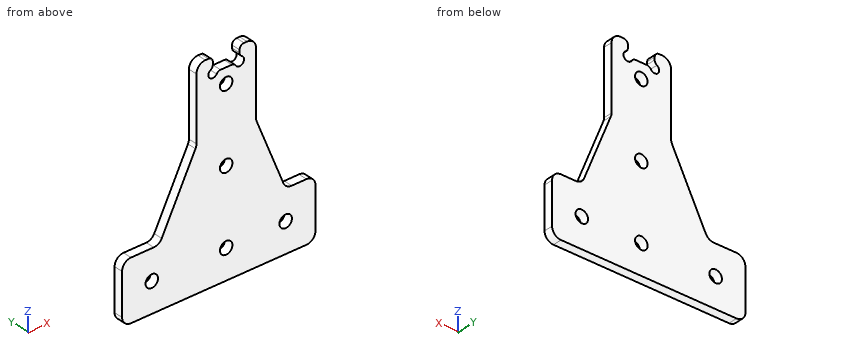
```python
from build123d import *

# Parameters (mm, degrees)
SKETCH_1_R          = 2.1
EXTRUDE_1_DEPTH     = 3
FILLET_1_R          = 3
SKETCH_2_W          = 9
SKETCH_2_H          = 5
CUT_EXTRUDE_1_DEPTH = 3
SKETCH_3_R          = 1.5
CUT_EXTRUDE_2_DEPTH = 10
FILLET_2_R          = 1.5


with BuildPart() as part:
    # 草图1 → 凸台-拉伸1 (new body)
    # profile 1 of 3: a face of its own
    with BuildSketch(Plane(origin=(0, 0, 0), x_dir=(1, 0, 0), z_dir=(0, 1, 0))):
        Polygon((10, -10), (30, -10), (30, 10), (-35, 10), (-35, -10), (-10, -10), (-10, -60), (10, -60), align=None)
        with Locations(Location((0, -50, 0), (0, 0, 270))):
            Circle(SKETCH_1_R, mode=Mode.SUBTRACT)
        with Locations(Location((0, -25, 0), (0, 0, 270))):
            Circle(SKETCH_1_R, mode=Mode.SUBTRACT)
        with Locations(Location((-25, 0, 0), (0, 0, 270))):
            Circle(SKETCH_1_R, mode=Mode.SUBTRACT)
        with Locations(Location((20, 0, 0), (0, 0, 270))):
            Circle(SKETCH_1_R, mode=Mode.SUBTRACT)
        with Locations(Location((0, 0, 0), (0, 0, 270))):
            Circle(SKETCH_1_R, mode=Mode.SUBTRACT)
    # profile 2 of 3: a face of its own
    with BuildSketch(Plane(origin=(0, 0, 0), x_dir=(1, 0, 0), z_dir=(0, 1, 0))):
        Polygon((-10, -10), (-22.5, -10), (-10, -35), align=None)
    # profile 3 of 3: a face of its own
    with BuildSketch(Plane(origin=(0, 0, 0), x_dir=(1, 0, 0), z_dir=(0, 1, 0))):
        Polygon((10, -35), (20, -10), (10, -10), align=None)
    extrude(amount=EXTRUDE_1_DEPTH)

    # 圆角1
    fillet_1_edges = [part.edges().sort_by_distance(p)[0] for p in [
        (10, 1.5, 35),
        (10, 1.5, 60),
        (-10, 1.5, 60),
        (-10, 1.5, 35),
        (-22.5, 1.5, 10),
        (-35, 1.5, 10),
        (-35, 1.5, -10),
        (30, 1.5, -10),
        (30, 1.5, 10),
        (20, 1.5, 10),
    ]]
    fillet(fillet_1_edges, radius=FILLET_1_R)

    # 草图2 → 切除-拉伸1 (cut)
    with BuildSketch(Plane(origin=(0, 3, 0), x_dir=(1, 0, 0), z_dir=(0, 1, 0))):
        with Locations((0, -57.5)):
            Rectangle(SKETCH_2_W, SKETCH_2_H)
    extrude(amount=-CUT_EXTRUDE_1_DEPTH, mode=Mode.SUBTRACT)

    # 草图3 → 切除-拉伸2 (cut)
    with BuildSketch(Plane(origin=(0, 3, 0), x_dir=(1, 0, 0), z_dir=(0, 1, 0))):
        with Locations((-4.5, -55)):
            Circle(SKETCH_3_R)
        with Locations((4.5, -55)):
            Circle(SKETCH_3_R)
    extrude(amount=-CUT_EXTRUDE_2_DEPTH, mode=Mode.SUBTRACT)

    # 圆角2
    fillet_2_edges = [part.edges().sort_by_distance(p)[0] for p in [
        (-4.5, 1.5, 60),
        (4.5, 1.5, 60),
        (4.5, 1.5, 56.5),
        (-3, 1.5, 55),
        (-4.5, 1.5, 56.5),
        (3, 1.5, 55),
    ]]
    fillet(fillet_2_edges, radius=FILLET_2_R)


solid = part.part
```
Can you work these out from the model? Positions are in its coordinate system, mm. Round coordinates to 2 decimals unless told otherwise and drop trailing zeros. Order: outer loops, then holes, each group sorted by start corner. A loop starts at its lowest first (then second) coordinate and runs counter-clockwise, first axis right, second up. Notation, with made-up numbers: (34.25, -4.75) -> (41.25, -4.75) arc R11 ccw to (41.25, 0.25) -> close; hole circle Ø1 at (-14, 63). An arc over 180 degrees is marked (long way). Return JSON: item names as keys, results as strings. Group by question number.
1. If we section it at C-C, the plane y = 1.1: Count the separate pieces of the cut face and the enclosed holes in it, then the cut area to 3 significant figures.
2. If we section it at A-A, the plane z = 0: Write out the boundary of the cut face in (x, y), then the cut area to 3 significant figures.
3. If we section it at D-D, the plane x = 23.5: Write out the boundary of the cut face in (y, z).
4. I need wall thicknesses on line 1 (X direction, y = 1.95, z = 0); line 2 (X direction, y = 2.8, z = 50); line 3 (Z direction, x = 12, y = 0.8). Which ranges of each line are inside material? Lowest first, please. Write a range as [from, to].
5. Will these pins go through, and if not, where does the flat tip stop? pin 1 (4 mm diameter, centred on x = 20, z = 0, fed in from -Y); pin 2 (1.5 mm diameter, centred on x = 24.5, y = 1, fed in from +Z); pin 3 (0.9 mm diameter, centred on y = 1.5, z = 45.5, fed in from -X).
6. If we section it at B-B, the plane z = 50: Write out the boundary of the cut face in (x, y), then the cut area to 3 significant figures.
Output values:
{
 "1": {"separate pieces": "1", "enclosed holes": "5", "area": "2,440 mm²"},
 "2": {"outline": "(-35, 0) -> (-27.1, 0) -> (-27.1, 3) -> (-35, 3) -> close; (-22.9, 0) -> (-2.1, 0) -> (-2.1, 3) -> (-22.9, 3) -> close; (2.1, 0) -> (17.9, 0) -> (17.9, 3) -> (2.1, 3) -> close; (22.1, 0) -> (30, 0) -> (30, 3) -> (22.1, 3) -> close", "area": "157 mm²"},
 "3": {"outline": "(0, -10) -> (3, -10) -> (3, 10) -> (0, 10) -> close"},
 "4": {"line 1": "[-35, -27.1], [-22.9, -2.1], [2.1, 17.9], [22.1, 30]", "line 2": "[-10, -2.1], [2.1, 10]", "line 3": "[-10, 30]"},
 "5": {"pin 1": "through", "pin 2": "z = 10", "pin 3": "x = -10"},
 "6": {"outline": "(-10, 0) -> (-2.1, 0) -> (-2.1, 3) -> (-10, 3) -> close; (2.1, 0) -> (10, 0) -> (10, 3) -> (2.1, 3) -> close", "area": "47.4 mm²"}
}
